Study the drawing (mm; zero at the part's minimum x, y, z) and answer. A direction names the side the tool comes from. Coordinates: 2 decimals unless noted, no trailing zeros. Loops run counter-clockwise (first coordinate to the right, second up) from the corner with the lowest first, then second, coordinate; pieces in that order, holes last. Notation, with made-up numbers: (-28.5, 58.25) -> (-9.5, 58.25) arc R18 cw to (-9.5, 81.25) -> close; hole circle Ø5 at (1, 88.25). An arc over 180 degrees is marked (long way). Answer as a JSON object with one key per item and string values. Group by question number.
Q1. The part is cut by section A-A on y = 3.5. Write down the section's boundary in (x, z), and give its area (3 significant figures).
Q2. For the marked faces 1, 2 and 3, determine the directions among +Z, -Z, +X, -X, +Y, -Y from which every point of the face is accessible in a straight line to the end or side of a thin tool.
Q3. The part is cut by section B-B on z = 39.5. Write down the section's boundary in (x, y).
Q4. Each of these flat-tipped pins is pushed along its axis until it touches: P1, Ø3, axis at x = 1.5, z = 34.5, coming from the +Y side; P2, Ø1.5, axis at y = 2, z = 8.5, coming from the +X side. Where does it stop, or does it pass through?
Q5. Straight lines are drawn through the part: line 1 along Z through (x, y) = (5.75, 3); line 2 along Y through (x, z) = (3.75, 33); line 3 along Y through (x, z) = (5.75, 21). For each, find the intervals that lie inside material, in ascending order. Write a range as [from, to].
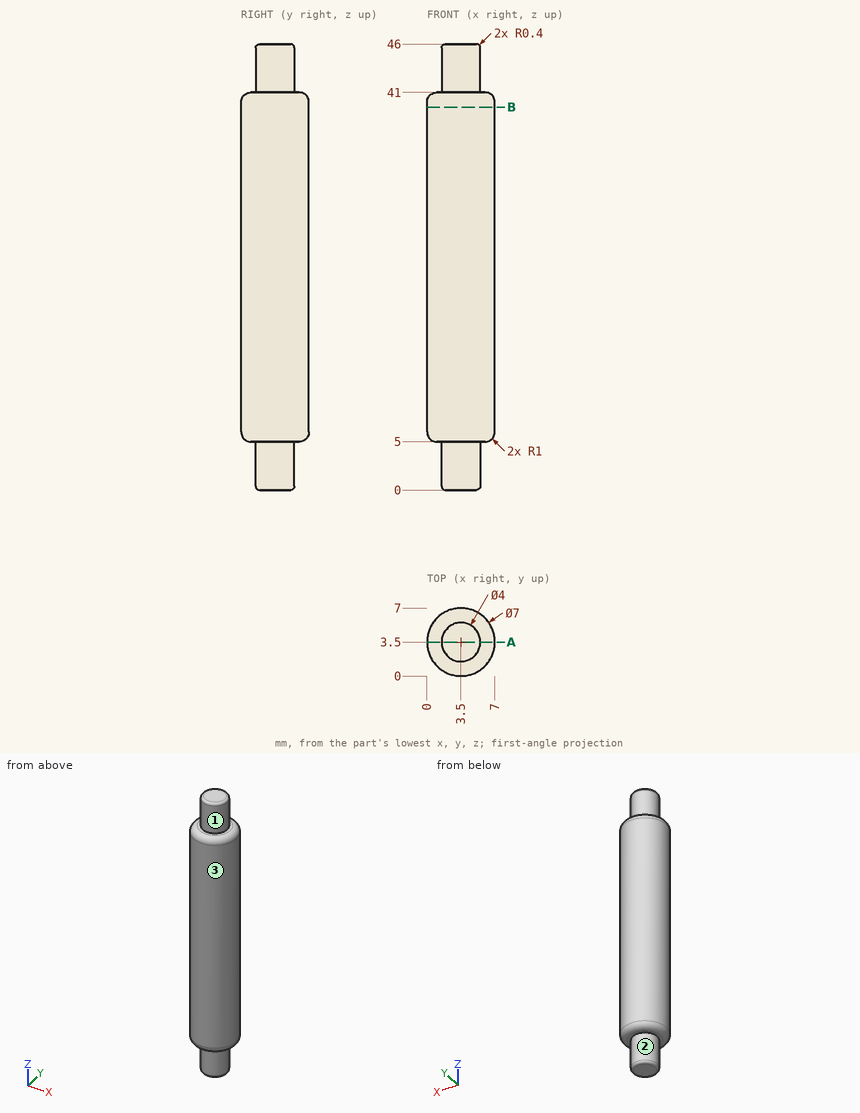
Final values:
{
 "1": {"outline": "(0, 6) arc R1 ccw to (1, 5) -> (1.5, 5) -> (1.5, 0.4) arc R0.4 ccw to (1.9, 0) -> (5.1, 0) arc R0.4 ccw to (5.5, 0.4) -> (5.5, 5) -> (6, 5) arc R1 ccw to (7, 6) -> (7, 40) arc R1 ccw to (6, 41) -> (5.5, 41) -> (5.5, 45.6) arc R0.4 ccw to (5.1, 46) -> (1.9, 46) arc R0.4 ccw to (1.5, 45.6) -> (1.5, 41) -> (1, 41) arc R1 ccw to (0, 40) -> close", "area": "291 mm2"},
 "2": {"face 1": "+Z", "face 2": "-Z", "face 3": "+Z, -Z"},
 "3": {"outline": "circle Ø7 at (3.5, 3.5)"},
 "4": {"P1": "stops at y = 6.96", "P2": "stops at x = 6.92"},
 "5": {"line 1": "z = [5, 41]", "line 2": "y = [0.01, 6.99]", "line 3": "y = [0.82, 6.18]"}
}
